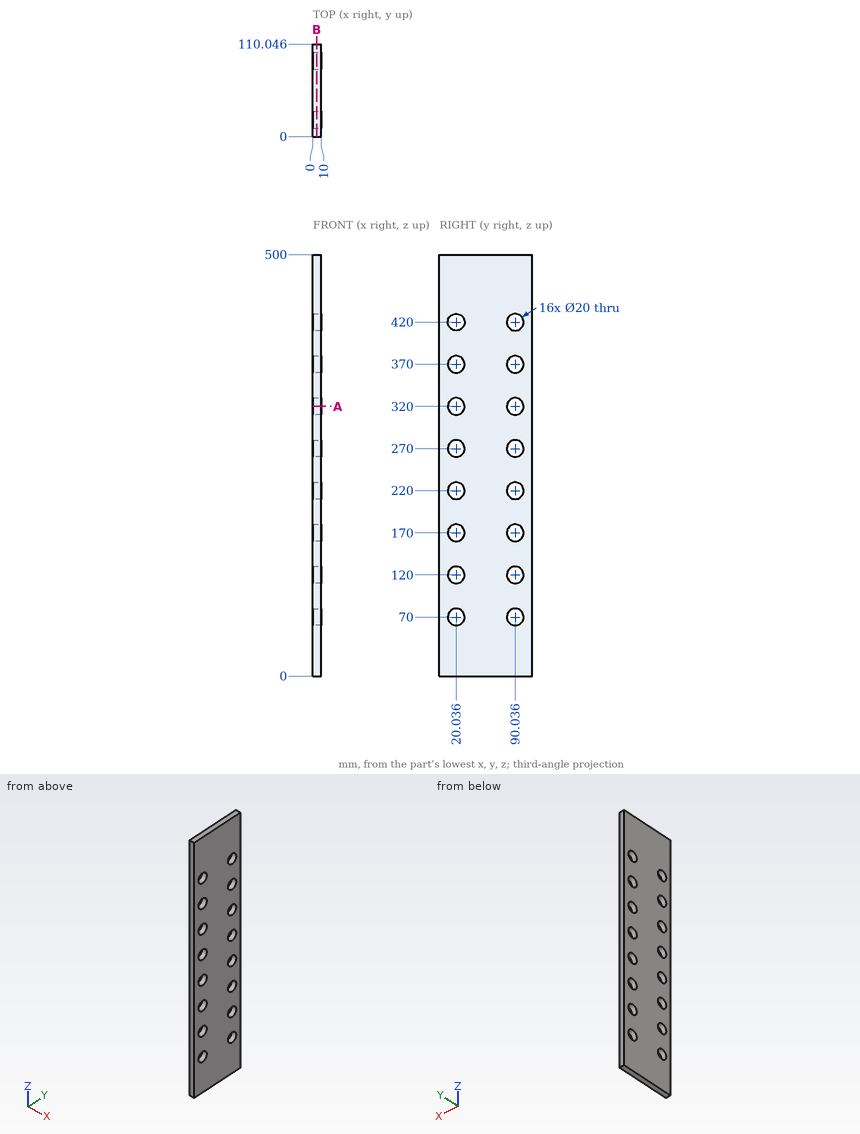
Part print with two shaded views. Sizes in mm from the minimum x, y, z corner. Coordinates: 2 decimals unless noted, no trailing zeros. Write each loop counter-clockwise with the first axis right and the second up, starting at its lowest first coordinate (ties: lowest second). Pieces come first, ordered by that corner, then holes. Notation, with made-up numbers: (2, -38) - (23, -38) arc R21 cw to (23, 0) - close; hole circle Ø4 at (-34.5, -34). An arc over 180 degrees is marked (long way). Put each result on its own line as item: value.
1. Flat gauge pin, fed straight in: pin 1 Ø23 at (y, z) = (20.04, 270) entering from -X. Where does the tip first touch, or does it go through?
Final values:
pin 1: stops at x = 0
2. Band-saw the part on A-A (z = 320). Write the cut outline in (x, y).
Final values:
outline: (0, 0) - (10, 0) - (10, 10.04) - (0, 10.04) - close; (0, 30.04) - (10, 30.04) - (10, 80.04) - (0, 80.04) - close; (0, 100.04) - (10, 100.04) - (10, 110.05) - (0, 110.05) - close
3. Probe line 1 along Y through (x, z) = (4.25, 120); line 2 along Y through (x, z) = (7.5, 327) (1 decimal). List the from-to ranges inside material, lowest first. Write a range as [from, to].
Final values:
line 1: y = [0, 10.04], [30.04, 80.04], [100.04, 110.05]
line 2: y = [0, 12.9], [27.2, 82.9], [97.2, 110]
4. Band-saw the part on B-B (x = 4.5). Give the number of separate pieces and of enclosed holes in the cut face, then the cut area to 3 significant figures.
Final values:
separate pieces: 1
enclosed holes: 16
area: 50,000 mm²
